Read the model definition and answer for the solid it produces. Units are mm, in the model's axes. Face numbers are marked on the shaded views. Give positions to 0.01 mm unless a question says otherwise; leave off trailing zeros. Write each loop counter-clockwise with the first axis right and the second up, starting at its lowest first coordinate (ties: lowest second). Pieces come first, ordered by that corner, then holes. Notation, with made-up numbers: (-29.5, 35) -> (-3.5, 35) arc R35 cw to (-3.5, 71) -> close; hole circle Ø10 at (-36.5, -37.75). An arc over 180 degrees is marked (long way). Put each result on its own line as item: value. Start each with the question number.
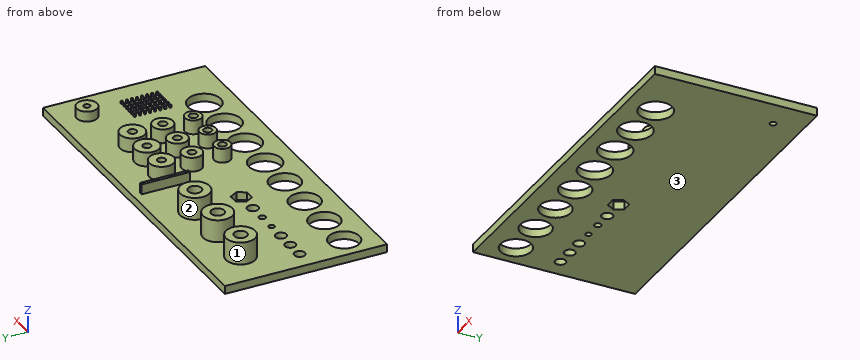
from build123d import *

# Parameters (mm, degrees)
SKETCH1_W            = 175
SKETCH1_H            = 80
SKETCH1_R            = 7.55
SKETCH1_R_2          = 7.575
SKETCH1_R_3          = 7.6
SKETCH1_R_4          = 7.625
SKETCH1_R_5          = 8.025
SKETCH1_R_6          = 8.05
SKETCH1_R_7          = 8.075
SKETCH1_R_8          = 8.1
SKETCH1_R_9          = 2.6
SKETCH1_R_10         = 2.65
SKETCH1_R_11         = 2.7
SKETCH1_R_12         = 1.45
SKETCH1_R_13         = 1.7
SKETCH1_R_14         = 2.75
BOSS_EXTRUDE1_DEPTH  = 4
SKETCH2_R            = 4
SKETCH2_R_2          = 2
BOSS_EXTRUDE2_DEPTH  = 7
SKETCH3_R            = 5
SKETCH3_R_2          = 2
BOSS_EXTRUDE3_DEPTH  = 7
SKETCH4_R            = 6
SKETCH4_R_2          = 2
BOSS_EXTRUDE4_DEPTH  = 7
SKETCH5_R            = 4.05
SKETCH5_R_2          = 2.05
BOSS_EXTRUDE5_DEPTH  = 7
SKETCH6_R            = 5.05
SKETCH6_R_2          = 2.05
BOSS_EXTRUDE6_DEPTH  = 7
SKETCH7_R            = 6.05
SKETCH7_R_2          = 2.05
BOSS_EXTRUDE7_DEPTH  = 7
SKETCH8_R            = 4.1
SKETCH8_R_2          = 2.1
BOSS_EXTRUDE8_DEPTH  = 7
SKETCH9_R            = 5.1
SKETCH9_R_2          = 2.1
BOSS_EXTRUDE9_DEPTH  = 7
SKETCH10_R           = 6.1
SKETCH10_R_2         = 2.1
BOSS_EXTRUDE10_DEPTH = 7
SKETCH11_R           = 7.2
SKETCH11_R_2         = 3.2
BOSS_EXTRUDE11_DEPTH = 11.1
SKETCH12_R           = 7.25
SKETCH12_R_2         = 3.25
BOSS_EXTRUDE12_DEPTH = 11.1
SKETCH13_R           = 7.3
SKETCH13_R_2         = 3.3
BOSS_EXTRUDE13_DEPTH = 11.1
SKETCH14_W           = 1.6
SKETCH14_H           = 24
BOSS_EXTRUDE14_DEPTH = 5
SKETCH15_R           = 0.5
BOSS_EXTRUDE15_DEPTH = 1.2
SKETCH16_R           = 1.6
CUT_EXTRUDE1_DEPTH   = 4
SKETCH17_R           = 5.05
SKETCH17_R_2         = 1.6
BOSS_EXTRUDE16_DEPTH = 5


with BuildPart() as part:
    # Sketch1 → Boss-Extrude1 (new body)
    with BuildSketch(Plane.XY.offset(300)):
        with Locations((387.5, 340)):
            Rectangle(SKETCH1_W, SKETCH1_H)
        with Locations((312, 315)):
            Circle(SKETCH1_R, mode=Mode.SUBTRACT)
        with Locations((331, 315)):
            Circle(SKETCH1_R_2, mode=Mode.SUBTRACT)
        with Locations((350, 315)):
            Circle(SKETCH1_R_3, mode=Mode.SUBTRACT)
        with Locations((369, 315)):
            Circle(SKETCH1_R_4, mode=Mode.SUBTRACT)
        with Locations((388, 315)):
            Circle(SKETCH1_R_5, mode=Mode.SUBTRACT)
        with Locations((407.5, 315)):
            Circle(SKETCH1_R_6, mode=Mode.SUBTRACT)
        with Locations((427, 315)):
            Circle(SKETCH1_R_7, mode=Mode.SUBTRACT)
        with Locations((446.5, 315)):
            Circle(SKETCH1_R_8, mode=Mode.SUBTRACT)
        with Locations((310, 338)):
            Circle(SKETCH1_R_9, mode=Mode.SUBTRACT)
        with Locations((319, 338)):
            Circle(SKETCH1_R_10, mode=Mode.SUBTRACT)
        with Locations((328, 338)):
            Circle(SKETCH1_R_11, mode=Mode.SUBTRACT)
        with Locations((337, 338)):
            Circle(SKETCH1_R_12, mode=Mode.SUBTRACT)
        with Locations((346, 338)):
            Circle(SKETCH1_R_13, mode=Mode.SUBTRACT)
        with Locations((355, 338)):
            Circle(SKETCH1_R_14, mode=Mode.SUBTRACT)
        Polygon((370.734272207, 338), (368.367136104, 342.1), (363.632863896, 342.1), (361.265727793, 338), (363.632863896, 333.9), (368.367136104, 333.9), align=None, mode=Mode.SUBTRACT)
    extrude(amount=BOSS_EXTRUDE1_DEPTH)

    # Sketch2 → Boss-Extrude2 (add)
    with BuildSketch(Plane.XY.offset(304)):
        with Locations((400, 330)):
            Circle(SKETCH2_R)
        with Locations((400, 330)):
            Circle(SKETCH2_R_2, mode=Mode.SUBTRACT)
    extrude(amount=BOSS_EXTRUDE2_DEPTH)

    # Sketch3 → Boss-Extrude3 (add)
    with BuildSketch(Plane.XY.offset(304)):
        with Locations((400, 345)):
            Circle(SKETCH3_R)
        with Locations((400, 345)):
            Circle(SKETCH3_R_2, mode=Mode.SUBTRACT)
    extrude(amount=BOSS_EXTRUDE3_DEPTH)

    # Sketch4 → Boss-Extrude4 (add)
    with BuildSketch(Plane.XY.offset(304)):
        with Locations((400, 360)):
            Circle(SKETCH4_R)
        with Locations((400, 360)):
            Circle(SKETCH4_R_2, mode=Mode.SUBTRACT)
    extrude(amount=BOSS_EXTRUDE4_DEPTH)

    # Sketch5 → Boss-Extrude5 (add)
    with BuildSketch(Plane.XY.offset(304)):
        with Locations((414, 330)):
            Circle(SKETCH5_R)
        with Locations((414, 330)):
            Circle(SKETCH5_R_2, mode=Mode.SUBTRACT)
    extrude(amount=BOSS_EXTRUDE5_DEPTH)

    # Sketch6 → Boss-Extrude6 (add)
    with BuildSketch(Plane.XY.offset(304)):
        with Locations((414, 345)):
            Circle(SKETCH6_R)
        with Locations((414, 345)):
            Circle(SKETCH6_R_2, mode=Mode.SUBTRACT)
    extrude(amount=BOSS_EXTRUDE6_DEPTH)

    # Sketch7 → Boss-Extrude7 (add)
    with BuildSketch(Plane.XY.offset(304)):
        with Locations((414, 360)):
            Circle(SKETCH7_R)
        with Locations((414, 360)):
            Circle(SKETCH7_R_2, mode=Mode.SUBTRACT)
    extrude(amount=BOSS_EXTRUDE7_DEPTH)

    # Sketch8 → Boss-Extrude8 (add)
    with BuildSketch(Plane.XY.offset(304)):
        with Locations((428, 330)):
            Circle(SKETCH8_R)
        with Locations((428, 330)):
            Circle(SKETCH8_R_2, mode=Mode.SUBTRACT)
    extrude(amount=BOSS_EXTRUDE8_DEPTH)

    # Sketch9 → Boss-Extrude9 (add)
    with BuildSketch(Plane.XY.offset(304)):
        with Locations((428, 345)):
            Circle(SKETCH9_R)
        with Locations((428, 345)):
            Circle(SKETCH9_R_2, mode=Mode.SUBTRACT)
    extrude(amount=BOSS_EXTRUDE9_DEPTH)

    # Sketch10 → Boss-Extrude10 (add)
    with BuildSketch(Plane.XY.offset(304)):
        with Locations((428, 360)):
            Circle(SKETCH10_R)
        with Locations((428, 360)):
            Circle(SKETCH10_R_2, mode=Mode.SUBTRACT)
    extrude(amount=BOSS_EXTRUDE10_DEPTH)

    # Sketch11 → Boss-Extrude11 (add)
    with BuildSketch(Plane.XY.offset(304)):
        with Locations((320, 362)):
            Circle(SKETCH11_R)
        with Locations((320, 362)):
            Circle(SKETCH11_R_2, mode=Mode.SUBTRACT)
    extrude(amount=BOSS_EXTRUDE11_DEPTH)

    # Sketch12 → Boss-Extrude12 (add)
    with BuildSketch(Plane.XY.offset(304)):
        with Locations((342, 362)):
            Circle(SKETCH12_R)
        with Locations((342, 362)):
            Circle(SKETCH12_R_2, mode=Mode.SUBTRACT)
    extrude(amount=BOSS_EXTRUDE12_DEPTH)

    # Sketch13 → Boss-Extrude13 (add)
    with BuildSketch(Plane.XY.offset(304)):
        with Locations((364, 362)):
            Circle(SKETCH13_R)
        with Locations((364, 362)):
            Circle(SKETCH13_R_2, mode=Mode.SUBTRACT)
    extrude(amount=BOSS_EXTRUDE13_DEPTH)

    # Sketch14 → Boss-Extrude14 (add)
    with BuildSketch(Plane.XY.offset(304)):
        with Locations((388.8, 364)):
            Rectangle(SKETCH14_W, SKETCH14_H)
    extrude(amount=BOSS_EXTRUDE14_DEPTH)

    # Sketch15 → Boss-Extrude15 (add)
    with BuildSketch(Plane.XY.offset(304)):
        with Locations((450, 330)):
            Circle(SKETCH15_R)
        with Locations((452.5, 330)):
            Circle(SKETCH15_R)
        with Locations((455, 330)):
            Circle(SKETCH15_R)
        with Locations((457.5, 330)):
            Circle(SKETCH15_R)
        with Locations((460, 330)):
            Circle(SKETCH15_R)
        with Locations((462.5, 330)):
            Circle(SKETCH15_R)
        with Locations((450, 332.5)):
            Circle(SKETCH15_R)
        with Locations((452.5, 332.5)):
            Circle(SKETCH15_R)
        with Locations((455, 332.5)):
            Circle(SKETCH15_R)
        with Locations((457.5, 332.5)):
            Circle(SKETCH15_R)
        with Locations((460, 332.5)):
            Circle(SKETCH15_R)
        with Locations((462.5, 332.5)):
            Circle(SKETCH15_R)
        with Locations((450, 335)):
            Circle(SKETCH15_R)
        with Locations((452.5, 335)):
            Circle(SKETCH15_R)
        with Locations((455, 335)):
            Circle(SKETCH15_R)
        with Locations((457.5, 335)):
            Circle(SKETCH15_R)
        with Locations((460, 335)):
            Circle(SKETCH15_R)
        with Locations((462.5, 335)):
            Circle(SKETCH15_R)
        with Locations((450, 337.5)):
            Circle(SKETCH15_R)
        with Locations((452.5, 337.5)):
            Circle(SKETCH15_R)
        with Locations((455, 337.5)):
            Circle(SKETCH15_R)
        with Locations((457.5, 337.5)):
            Circle(SKETCH15_R)
        with Locations((460, 337.5)):
            Circle(SKETCH15_R)
        with Locations((462.5, 337.5)):
            Circle(SKETCH15_R)
        with Locations((450, 340)):
            Circle(SKETCH15_R)
        with Locations((452.5, 340)):
            Circle(SKETCH15_R)
        with Locations((455, 340)):
            Circle(SKETCH15_R)
        with Locations((457.5, 340)):
            Circle(SKETCH15_R)
        with Locations((460, 340)):
            Circle(SKETCH15_R)
        with Locations((462.5, 340)):
            Circle(SKETCH15_R)
        with Locations((450, 342.5)):
            Circle(SKETCH15_R)
        with Locations((452.5, 342.5)):
            Circle(SKETCH15_R)
        with Locations((455, 342.5)):
            Circle(SKETCH15_R)
        with Locations((457.5, 342.5)):
            Circle(SKETCH15_R)
        with Locations((460, 342.5)):
            Circle(SKETCH15_R)
        with Locations((462.5, 342.5)):
            Circle(SKETCH15_R)
        with Locations((450, 345)):
            Circle(SKETCH15_R)
        with Locations((452.5, 345)):
            Circle(SKETCH15_R)
        with Locations((455, 345)):
            Circle(SKETCH15_R)
        with Locations((457.5, 345)):
            Circle(SKETCH15_R)
        with Locations((460, 345)):
            Circle(SKETCH15_R)
        with Locations((462.5, 345)):
            Circle(SKETCH15_R)
        with Locations((450, 347.5)):
            Circle(SKETCH15_R)
        with Locations((452.5, 347.5)):
            Circle(SKETCH15_R)
        with Locations((455, 347.5)):
            Circle(SKETCH15_R)
        with Locations((457.5, 347.5)):
            Circle(SKETCH15_R)
        with Locations((460, 347.5)):
            Circle(SKETCH15_R)
        with Locations((462.5, 347.5)):
            Circle(SKETCH15_R)
    extrude(amount=BOSS_EXTRUDE15_DEPTH)

    # Sketch16 → Cut-Extrude1 (cut)
    with BuildSketch(Plane.XY.offset(300)):
        with Locations((460, 366)):
            Circle(SKETCH16_R)
    extrude(amount=CUT_EXTRUDE1_DEPTH, mode=Mode.SUBTRACT)

    # Sketch17 → Boss-Extrude16 (add)
    with BuildSketch(Plane.XY.offset(304)):
        with Locations((460, 366)):
            Circle(SKETCH17_R)
        with Locations((460, 366)):
            Circle(SKETCH17_R_2, mode=Mode.SUBTRACT)
    extrude(amount=BOSS_EXTRUDE16_DEPTH)


solid = part.part
1) For a pull along X with two mould halves and no side action, classify the marked faces 1, 2 and 3 as pulls with the +X half, pulls with the -X half, needs draft (parallel to the pull), parting line crosses it, or undercut.
2) Each of these flat-tipped pins is pushed along its axis until it touches: pin 1 Ø1.1 at (x, y) = (450, 332.5) entering from +Z; pin 2 Ø3 at (y, z) = (345.5, 306.5) entering from +X; pin 3 Ø5 at (x, y) = (328, 338) entering from -Z; pin 4 Ø10 at (x, y) = (432, 312.5) entering from -Z. Where does it stop, or does it pass through?
3) A cutting plane is placed at A-A on x = 310. Give the vertices of the cut face in (y, z).
4) A cutting plane is placed at D-D on x = 355. Give the vertices of the cut face in (y, z), and give its area (3 significant figures).
5) A cutting plane is placed at C-C on y = 305. Give the vertices of the cut face in (x, z).
6) A cutting plane is placed at B-B on x = 382. Give the vertices of the cut face in (y, z), and give its area (3 significant figures).
7) Straight lines are drawn through the part: line 1 (Y direction, x = 428, z = 306.75); line 2 (Y direction, x = 414, z = 307.25); line 3 (X direction, y = 357.5, z = 310.5). For each, find the intervals that lie inside material, in ascending order. Write a range as [from, to].
Results found:
1. face 1: undercut
1. face 2: undercut
1. face 3: needs draft
2. pin 1: stops at z = 305.2
2. pin 2: stops at x = 463
2. pin 3: passes through
2. pin 4: stops at z = 300
3. outline: (300, 300) -> (307.72, 300) -> (307.72, 304) -> (300, 304) -> close; (322.28, 300) -> (335.4, 300) -> (335.4, 304) -> (322.28, 304) -> close; (340.6, 300) -> (380, 300) -> (380, 304) -> (340.6, 304) -> close
4. outline: (300, 300) -> (309.28, 300) -> (309.28, 304) -> (300, 304) -> close; (320.72, 300) -> (335.25, 300) -> (335.25, 304) -> (320.72, 304) -> close; (340.75, 300) -> (380, 300) -> (380, 304) -> (340.75, 304) -> close
4. area: 252 mm²
5. outline: (300, 300) -> (475, 300) -> (475, 304) -> (300, 304) -> close
6. outline: (300, 300) -> (309.67, 300) -> (309.67, 304) -> (300, 304) -> close; (320.33, 300) -> (380, 300) -> (380, 304) -> (320.33, 304) -> close
6. area: 277 mm²
7. line 1: y = [325.9, 327.9], [332.1, 334.1], [339.9, 342.9], [347.1, 350.1], [353.9, 357.9], [362.1, 366.1]
7. line 2: y = [325.95, 327.95], [332.05, 334.05], [339.95, 342.95], [347.05, 350.05], [353.95, 357.95], [362.05, 366.05]
7. line 3: x = [314.38, 325.62], [336.32, 347.68], [358.25, 369.75], [394.55, 405.45], [408.49, 419.51], [422.44, 433.56]
